from build123d import *

# Parameters (mm, degrees)
BOSS_EXTRUDE1_DEPTH  = 1.5875
M3_CLEARANCE_HOLE1_D = 3.4
M3_CLEARANCE_HOLE2_D = 3.4
CIRPATTERN1_COUNT    = 8
FILLET1_R            = 5.08


with BuildPart() as part:
    # Sketch1 → Boss-Extrude1 (new, symmetric)
    with BuildSketch(Plane(origin=(0, 0, 0), x_dir=(1, 0, 0), z_dir=(0, 1, 0))):
        with BuildLine():
            Line((-38.50947489, 32.14883464), (-38.50947489, -32.14883464))
            ThreePointArc((-38.50947489, -32.14883464), (-35.992876625, -34.943383598), (-33.274, -37.541552299))
            Line((-33.274, -37.541552299), (33.274, -37.541552299))
            ThreePointArc((33.274, -37.541552299), (36.035191498, -34.899744966), (38.587271968, -32.055415565))
            Line((38.587271968, -32.055415565), (4.572, -9.720985565))
            Line((4.572, -9.720985565), (4.572, 9.720985565))
            Line((4.572, 9.720985565), (38.541369471, 32.110591154))
            ThreePointArc((38.541369471, 32.110591154), (35.567819018, 35.375944868), (32.318597457, 38.367114609))
            Line((32.318597457, 38.367114609), (-32.318597457, 38.367114609))
            ThreePointArc((-32.318597457, 38.367114609), (-35.55025611, 35.393594272), (-38.50947489, 32.14883464))
        make_face()
    extrude(amount=BOSS_EXTRUDE1_DEPTH, both=True)

    # M3 Clearance Hole1 (through all)
    with Locations(Plane(origin=(0, 1.5875, 0), x_dir=(1, 0, 0), z_dir=(0, 1, 0))):
        with Locations((-33.226947648, 33.226947648), (33.226947648, 33.226947648), (33.226947648, -33.226947648), (-33.226947648, -33.226947648)):
            Hole(M3_CLEARANCE_HOLE1_D / 2)

    # M3 Clearance Hole2 (through all)
    with Locations(Plane(origin=(0, -1.5875, 0), x_dir=(-1, 0, 0), z_dir=(0, -1, 0))):
        with Locations((4.66144561, -4.592201188)):
            m3_clearance_hole2 = Hole(M3_CLEARANCE_HOLE2_D / 2)

    # CirPattern1: M3 Clearance Hole2 ×8 about axis
    cirpattern1_axis = Axis((-15.748, 0, 0), (0, 1, 0))
    for i in range(1, CIRPATTERN1_COUNT):
        add(m3_clearance_hole2.rotate(cirpattern1_axis, i * 360 / CIRPATTERN1_COUNT), mode=Mode.SUBTRACT)

    # Fillet1
    fillet1_edges = [part.edges().sort_by_distance(p)[0] for p in [
        (4.572, 0, -9.720985565),
        (4.572, 0, 9.720985565),
    ]]
    fillet(fillet1_edges, radius=FILLET1_R)


solid = part.part
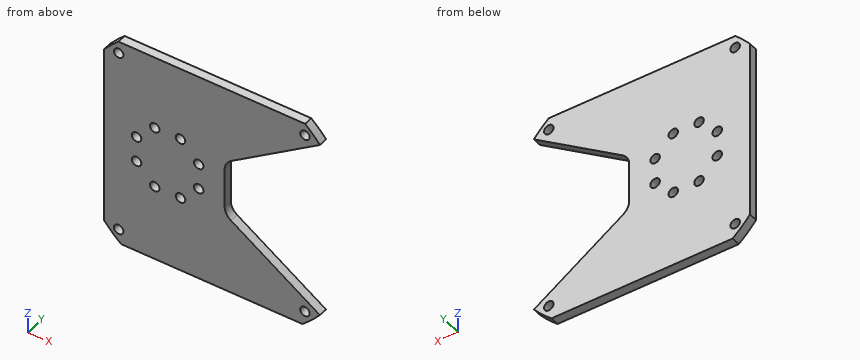
Source: CAD feature listing. Evaluate the final solid. Frame: model axes, mm. Coordinates: 2 decimals unless noted, no trailing zeros. Order: outer loops, then holes, each group sorted by start corner. A loop starts at its lowest first (then second) coordinate and runs counter-clockwise, first axis right, second up. Notation, with made-up numbers: M 45.5,-1.5 L 62.5,-1.5 A25 cw 62.5,37.5 Z; hole C -36,-30 d3. An arc over 180 degrees is marked long. Write each question's results on one line, items separated by ' | '. Start each with the question number.
1. Material intervals for L1, parallel to Z at x = -5.5, y = 0.6; L2, parallel to X at y = 0.8, z = -12.5; L3, parallel to Z at x = 32, y = 1.45, sorted ascending.
2. Section C-C, the plane z = -17. Return the cut outline in (x, y).
3. Pin query (flat end, axial travel): pin 1 (3 mm diameter, centred on x = -26.83, z = -4.59, fed in from -Y). Return the tip coordinate at first contact, or that it passes through.
4. Section A-A, the plane x = 28. Return the cut outline in (y, z).
5. Section B-B, the plane y = -0.35. State how many separate pieces and enclosed holes the cut face has, then the cut area to 3 significant figures.
6. Section D-D, the plane z = 22. Return the cut outline in (x, y), then the cut area to 3 significant figures.
Solution:
1) L1: -38.37 to -6.07, -3.11 to 3.11, 6.07 to 37.54 | L2: -38.51 to -21.28, -19.4 to -12.1, -10.21 to 8.79 | L3: -38.37 to -34.4, -32.05 to -27.8, 27.73 to 32.05, 34.4 to 37.54
2) outline: M -38.51,-1.59 L 15.62,-1.59 L 15.62,1.59 L -38.51,1.59 Z
3) pin 1: through
4) outline: M -1.59,-38.37 L 1.59,-38.37 L 1.59,-25.16 L -1.59,-25.16 Z; M -1.59,25.1 L 1.59,25.1 L 1.59,37.54 L -1.59,37.54 Z
5) separate pieces: 1 | enclosed holes: 12 | area: 4,260 mm²
6) outline: M -38.51,-1.59 L 23.27,-1.59 L 23.27,1.59 L -38.51,1.59 Z | area: 196 mm²
